Read the model definition and answer for the solid it produces. Units are mm, in the model's axes. Coordinates: 2 decimals unless noted, no trailing zeros. Order: outer loops, then holes, each group sorted by start corner. A loop starts at its lowest first (then second) coordinate and runs counter-clockwise, first axis right, second up. Notation, with made-up numbers: (-3, 10.25) -> (2, 10.25) arc R30 cw to (2, 41.25) -> close; hole circle Ø6 at (-35.75, -8.75). An arc over 180 degrees is marked (long way). Answer as a JSON object with one key per item and string values. Group by question number.
1) Consider L1, parallel to Z at x = 0.75, y = 77; L2, parallel to Z at x = 1.2, y = 7; L3, parallel to Y at x = 0.35, z = 13. Determine where each line is inside the solid, lowest interval first.
2) Determine the mould class of faces 1 (the flat face through (-1.5, 38, -10)), 2 (the cylindrical face through (0.02, 22.19, -35.09)), 3 (the flat face through (0.021, 64.852, -32.235)), 4 (the flat face through (0.021, 70.887, -9.674)) for opening direction Y: released by +Y, released by -Y, zero draft, split by the parting line, or undercut.
3) Section B-B on y = 47 is taken. Determine the outline of the cut face in (x, z), and give its area (3 significant figures).
4) Section A-A on y = 21 is taken. Determine the outline of the cut face in (x, z), and give its area (3 significant figures).
5) Given pin 1 (1.5 mm diameter, centred on x = -0.5, y = 35.5, fed in from -Z); pin 2 (1 mm diameter, centred on x = 0.5, y = 41, fed in from -Z); pin 3 (1 mm diameter, centred on x = 1, y = 10, fed in from +Z), each flat-ended and moving along its own axis, determine where each tip first touches the part or whether it passes through.
from build123d import *

# Parameters (mm, degrees)
BOSS_EXTRUDE1_DEPTH = 1.5


with BuildPart() as part:
    # Sketch1 (on Right Plane) → Boss-Extrude1 (new body, symmetric)
    with BuildSketch(Plane(origin=(0, 0, 0), x_dir=(0, 0, -1), z_dir=(1, 0, 0))):
        with BuildLine():
            Line((41.140439709, 94.354710036), (23.076518975, 34.512005167))
            ThreePointArc((23.076518975, 34.512005167), (35.21800412, 21.984003604), (41.140439709, 5.573907889))
            add(Edge.make_bspline(
                [(-41.516312801, 0), (0.187936546, -2.786953944), (41.140439709, 5.573907889)],
                knots=[0, 0, 0, 1, 1, 1], degree=2))
            ThreePointArc((-41.516312801, 0), (-29.070108459, 29.640057739), (0.805992023, 41.508488355))
            Line((0.805992023, 41.508488355), (18.79411763, 101.100096824))
            Line((18.79411763, 101.100096824), (41.140439709, 94.354710036))
        make_face()
    extrude(amount=BOSS_EXTRUDE1_DEPTH, both=True)


solid = part.part
Worked answers:
{
 "1": {"L1": "z = -35.9 to -11.52", "L2": "z = -40.92 to 40.92", "L3": "y = -0.6 to 39.43"},
 "2": {"face 1": "zero draft", "face 2": "undercut", "face 3": "undercut", "face 4": "released by +Y"},
 "3": {"outline": "(-1.5, -26.85) -> (1.5, -26.85) -> (1.5, -2.46) -> (-1.5, -2.46) -> close", "area": "73.1 mm²"},
 "4": {"outline": "(-1.5, -35.81) -> (1.5, -35.81) -> (1.5, 35.81) -> (-1.5, 35.81) -> close", "area": "215 mm²"},
 "5": {"pin 1": "stops at z = -23.6", "pin 2": "stops at z = -25.19", "pin 3": "stops at z = 40.41"}
}
